Model file for the job. Use its own axes, mm. Face numbers are marked on the shaded views. A direction names the side the tool comes from. Give positions to 0.01 mm unless a question says otherwise; leave off trailing zeros. Write each loop counter-clockwise with the first axis right and the second up, starting at its lowest first coordinate (ties: lowest second). Pieces come first, ordered by that corner, then holes. Notation, with made-up numbers: (12, 19.5) - (21, 19.5) arc R27 ccw to (21, 40.5) - close; hole circle Ø5 at (-8.75, -24). An arc over 180 degrees is marked (long way). One line per item, written item: value. Start each with the question number.
(1) 3-axis set-ups, long thin cutter, end or side, ignore diameter. For the marked faces 5, 6 and 7: which of +Z, -Z, +X, -X, +Y, -Y reach the whole face in a straight line?
(2) Probe L1, parallel to Y at x = -0.25, z = -7; L2, parallel to X at y = 48, z = 0.25; L3, parallel to Z at x = 1.25, y = 49.5. List the from-to ranges inside material, lowest first.
(3) Drop flat-ended pins along their axis: P1, Ø10, axis at x = -2.5, z = 8.5, coming from the +Y side; P2, Ø10, axis at x = 5, y = 41.5, coming from the +Z side; P3, Ø1.5, axis at x = 0.5, y = 55.5, coming from the -Z side; P4, Ø0.6, axis at x = -1.5, z = -3, coming from the +Y side. Give the stop position or say it passes through.
(4) Cut at A-A, the plane y = 32. List the corners of the cut face in (x, z).
(5) Mould opens along Y. For the marked faces 1, 2, 3 and 4 say: pulls with the +Y half, pulls with the -Y half, needs draft (parallel to the pull), parting line crosses it, or undercut.
from build123d import *

# Parameters (mm, degrees)
SKETCH1_RX          = 12.25
SKETCH1_RY          = 3.75
BOSS_EXTRUDE1_DEPTH = 1.5
SKETCH2_R           = 3.75
BOSS_EXTRUDE2_DEPTH = 58
SKETCH3_W           = 7.5
SKETCH3_H           = 15
CUT_EXTRUDE1_DEPTH  = 1
SKETCH4_W           = 12.491636394
SKETCH4_H           = 7.5
CUT_EXTRUDE2_DEPTH  = 1
CIRPATTERN1_COUNT   = 2


with BuildPart() as part:
    # Sketch1 → Boss-Extrude1 (new body)
    with BuildSketch(Plane(origin=(0, 0, 0), x_dir=(1, 0, 0), z_dir=(0, 1, 0))):
        with Locations((0, 0)):
            Ellipse(SKETCH1_RX, SKETCH1_RY)
        with Locations(Location((0, 0), (0, 0, 90))):
            Ellipse(SKETCH1_RX, SKETCH1_RY)
    extrude(amount=BOSS_EXTRUDE1_DEPTH)

    # Sketch2 → Boss-Extrude2 (add)
    with BuildSketch(Plane(origin=(0, 1.5, 0), x_dir=(1, 0, 0), z_dir=(0, 1, 0))):
        Circle(SKETCH2_R)
    extrude(amount=BOSS_EXTRUDE2_DEPTH)

    # Sketch3 → Cut-Extrude1 (cut)
    with BuildSketch(Plane.XY.offset(3.75)):
        with Locations((0, 52)):
            Rectangle(SKETCH3_W, SKETCH3_H)
    cut_extrude1 = extrude(amount=-CUT_EXTRUDE1_DEPTH, mode=Mode.SUBTRACT)

    # Sketch4 → Cut-Extrude2 (cut)
    with BuildSketch(Plane.XY.offset(2.75)):
        with Locations((0.147803462, 48.25)):
            Rectangle(SKETCH4_W, SKETCH4_H)
    cut_extrude2 = extrude(amount=-CUT_EXTRUDE2_DEPTH, mode=Mode.SUBTRACT)

    # CirPattern1: Cut-Extrude1, Cut-Extrude2 ×2 about axis
    cirpattern1_axis = Axis((0, 59.5, 0), (0, 1, 0))
    for i in range(1, CIRPATTERN1_COUNT):
        add(cut_extrude1.rotate(cirpattern1_axis, i * 360 / CIRPATTERN1_COUNT), mode=Mode.SUBTRACT)
        add(cut_extrude2.rotate(cirpattern1_axis, i * 360 / CIRPATTERN1_COUNT), mode=Mode.SUBTRACT)


solid = part.part
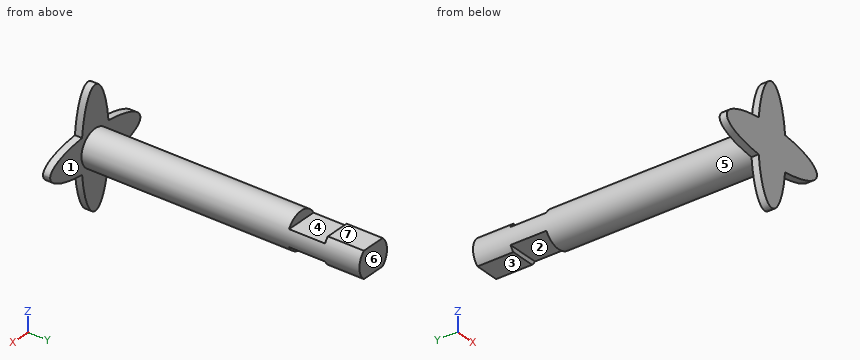
Answers follow:
1. face 5: +Y
1. face 6: +Z, -Z, +X, -X, +Y
1. face 7: +Z, +X, -X, +Y
2. L1: y = 0 to 1.5
2. L2: x = -3.74 to 3.74
2. L3: z = -1.75 to 1.75
3. P1: stops at y = 1.5
3. P2: stops at z = 3.75
3. P3: stops at z = -2.75
3. P4: stops at y = 59.5
4. outline: circle Ø7.5 at (0, 0)
5. face 1: pulls with the +Y half
5. face 2: undercut
5. face 3: needs draft
5. face 4: undercut
